Read the model definition and answer for the solid it produces. Units are mm, in the model's axes. Give positions to 0.01 mm unless a question says otherwise; leave off trailing zeros. Write each loop counter-clockwise with the first axis right and the second up, starting at its lowest first coordinate (ties: lowest second). Pieces come first, ordered by that corner, then holes.
```python
from build123d import *

# Parameters (mm, degrees)
SKETCH_1_R               = 25
EXTRUDE_1_DEPTH          = 3
CHAMFER_1_SIZE           = 1
SKETCH_2_R               = 2.75
CUT_EXTRUDE_1_DEPTH      = 36.482389998
PATTERN_CIRCULAR_1_COUNT = 4


with BuildPart() as part:
    # 草图1 → 凸台-拉伸1 (new body)
    with BuildSketch(Plane.XY):
        Circle(SKETCH_1_R)
    extrude(amount=EXTRUDE_1_DEPTH)

    # 倒角1
    chamfer_1_edges = [part.edges().sort_by_distance(p)[0] for p in [
        (-25, 0, 3),
    ]]
    chamfer(chamfer_1_edges, length=CHAMFER_1_SIZE)

    # 草图2 → 切除-拉伸1 (cut, through all)
    with BuildSketch(Plane.XY.offset(3)):
        with Locations((0, 20)):
            Circle(SKETCH_2_R)
    cut_extrude_1 = extrude(amount=-CUT_EXTRUDE_1_DEPTH, mode=Mode.SUBTRACT)

    # 阵列(圆周)1: 切除-拉伸1 ×4 about axis
    pattern_circular_1_axis = Axis((0, 0, 0), (0, 0, 1))
    for i in range(1, PATTERN_CIRCULAR_1_COUNT):
        add(cut_extrude_1.rotate(pattern_circular_1_axis, i * 360 / PATTERN_CIRCULAR_1_COUNT), mode=Mode.SUBTRACT)


solid = part.part
```
Item 1: Find the intervals of material crossed by line 1 along Y through (x, z) = (0, 0.6); line 2 along X through (y, z) = (2, 1.25); line 3 along Y through (x, z) = (-20, 0.7), in increasing order.
Result set:
line 1: y = -25 to -22.75, -17.25 to 17.25, 22.75 to 25
line 2: x = -24.92 to -21.89, -18.11 to 18.11, 21.89 to 24.92
line 3: y = -15 to -2.75, 2.75 to 15
Item 2: Section A-A (x = 0) is taken. Write down the section's boundary in (y, z).
Result set:
outline: (-25, 0) - (-22.75, 0) - (-22.75, 3) - (-24, 3) - (-25, 2) - close; (-17.25, 0) - (17.25, 0) - (17.25, 3) - (-17.25, 3) - close; (22.75, 0) - (25, 0) - (25, 2) - (24, 3) - (22.75, 3) - close
Item 3: Determine the mould class of faces 1 (the cylindrical face through (-22.727, -0.358, 1.521)), 2 (the cylindrical face through (-0.358, 22.727, 1.521)), 3 (the cylindrical face through (23.846, 7.509, 0.986)), 4 (the flat face through (0, 0, 0)) for opening direction Y: pulls with the +Y half, pulls with the -Y half, needs draft (parallel to the pull), parting line crosses it, or undercut.
Result set:
face 1: undercut
face 2: undercut
face 3: parting line crosses it
face 4: needs draft
Item 4: Section B-B (z = 0.9) is taken. Write down the section's boundary in (x, y), and give its area (3 significant figures).
Result set:
outline: circle Ø50 at (0, 0); hole circle Ø5.5 at (-20, 0); hole circle Ø5.5 at (0, -20); hole circle Ø5.5 at (0, 20); hole circle Ø5.5 at (20, 0)
area: 1,870 mm2
Item 5: Each of these flat-tipped pins is pushed along its axis until it touches: pin 1 Ø1 at (x, z) = (16, 1) entering from +Y; pin 2 Ø1.5 at (y, z) = (-12, 1) entering from -X; pin 3 Ø3.5 at (x, y) = (0, 20) entering from +Z. Where does it stop, or does it pass through?
Result set:
pin 1: stops at y = 19.62
pin 2: stops at x = -22.33
pin 3: passes through
